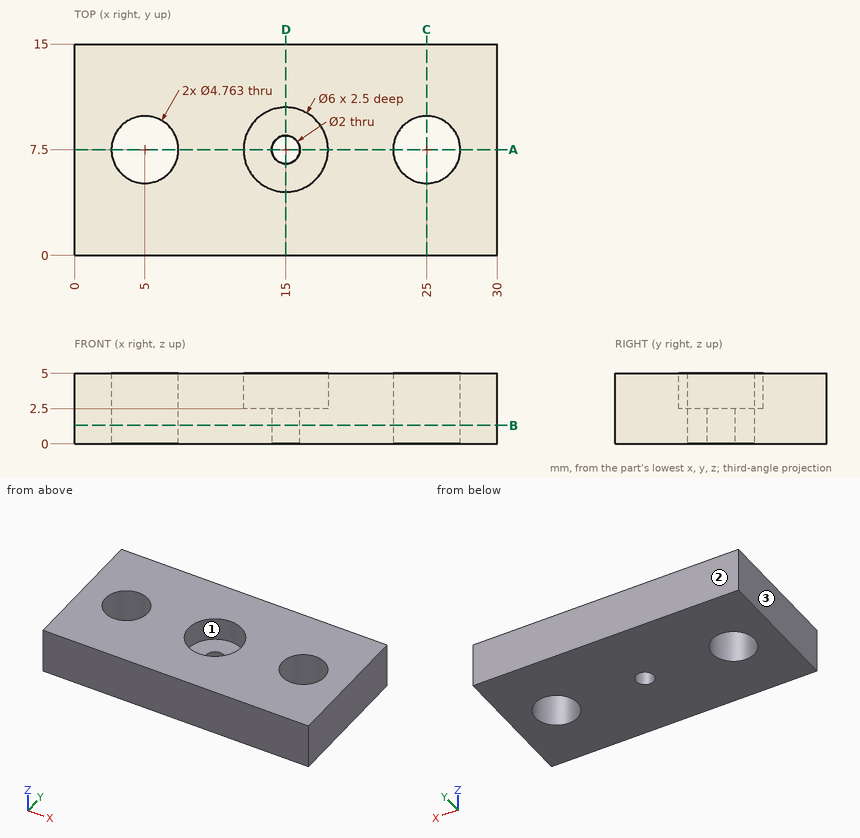
Study the drawing (mm; zero at the part's minimum x, y, z) and answer. Round coordinates to 2 decimals unless told otherwise and drop trailing zeros. Write each loop counter-clockwise with the first axis right and the second up, starting at its lowest first coordinate (ties: lowest second). Pieces come first, ordered by that corner, then holes.
1) Determine the mould class of the marked faces 1, 2 and 3 for opening direction X: pulls with the +X half, pulls with the -X half, needs draft (parallel to the pull), parting line crosses it, or undercut.
2) A cutting plane is placed at C-C on x = 25. Determine the outline of the cut face in (y, z).
3) A cutting plane is placed at D-D on x = 15. Determine the outline of the cut face in (y, z).
4) A cutting plane is placed at B-B on z = 1.3. Determine the outline of the cut face in (x, y).
5) A cutting plane is placed at A-A on y = 7.5. Determine the outline of the cut face in (x, z).
6) Consider probe 1 along X at (y, z) = (5.5, 3.65) (1 decimal); probe 2 along X at (y, z) = (8.5, 4.3); probe 3 along Y at (x, z) = (15, 3.1). Determine where each line is inside the solid, lowest interval first.
Entries:
1. face 1: undercut
1. face 2: needs draft
1. face 3: pulls with the -X half
2. outline: (0, 0) - (5.12, 0) - (5.12, 5) - (0, 5) - close; (9.88, 0) - (15, 0) - (15, 5) - (9.88, 5) - close
3. outline: (0, 0) - (6.5, 0) - (6.5, 2.5) - (4.5, 2.5) - (4.5, 5) - (0, 5) - close; (8.5, 0) - (15, 0) - (15, 5) - (10.5, 5) - (10.5, 2.5) - (8.5, 2.5) - close
4. outline: (0, 0) - (30, 0) - (30, 15) - (0, 15) - close; hole circle Ø4.76 at (5, 7.5); hole circle Ø2 at (15, 7.5); hole circle Ø4.76 at (25, 7.5)
5. outline: (0, 0) - (2.62, 0) - (2.62, 5) - (0, 5) - close; (7.38, 0) - (14, 0) - (14, 2.5) - (12, 2.5) - (12, 5) - (7.38, 5) - close; (16, 0) - (22.62, 0) - (22.62, 5) - (18, 5) - (18, 2.5) - (16, 2.5) - close; (27.38, 0) - (30, 0) - (30, 5) - (27.38, 5) - close
6. probe 1: x = 0 to 3.7, 6.3 to 12.8, 17.2 to 23.7, 26.3 to 30
6. probe 2: x = 0 to 2.84, 7.16 to 12.17, 17.83 to 22.84, 27.16 to 30
6. probe 3: y = 0 to 4.5, 10.5 to 15
